```python
from build123d import *

# Parameters (mm, degrees)
SKETCH3_W           = 19.70074215
SKETCH3_H           = 14.68
SKETCH3_R           = 2
BOSS_EXTRUDE2_DEPTH = 4
SKETCH5_W           = 4
SKETCH5_H           = 14.68
BOSS_EXTRUDE3_DEPTH = 20
SKETCH6_R           = 2
CUT_EXTRUDE1_DEPTH  = 10
FILLET1_R           = 2


with BuildPart() as part:
    # Sketch3 → Boss-Extrude2 (new body)
    with BuildSketch(Plane(origin=(0, 0, 0), x_dir=(1, 0, 0), z_dir=(0, 1, 0))):
        with Locations((0.919743343, 1.910780827)):
            Rectangle(SKETCH3_W, SKETCH3_H)
        with Locations((1.919743345, 1.910780827)):
            Circle(SKETCH3_R, mode=Mode.SUBTRACT)
    extrude(amount=BOSS_EXTRUDE2_DEPTH)

    # Sketch5 → Boss-Extrude3 (add)
    with BuildSketch(Plane(origin=(0, 4, 0), x_dir=(1, 0, 0), z_dir=(0, 1, 0))):
        with Locations((-6.930627732, 1.910780827)):
            Rectangle(SKETCH5_W, SKETCH5_H)
    extrude(amount=BOSS_EXTRUDE3_DEPTH)

    # Sketch6 → Cut-Extrude1 (cut)
    with BuildSketch(Plane(origin=(-4.930627732, 0, 0), x_dir=(0, 0, -1), z_dir=(1, 0, 0))):
        with Locations((1.910780827, 14)):
            Circle(SKETCH6_R)
    extrude(amount=-CUT_EXTRUDE1_DEPTH, mode=Mode.SUBTRACT)

    # Fillet1
    fillet1_edges = [part.edges().sort_by_distance(p)[0] for p in [
        (-4.930627732, 4, -1.910780827),
        (-6.930627732, 24, 5.429219173),
        (-6.930627732, 24, -9.250780827),
        (10.770114418, 2, -9.250780827),
        (10.770114418, 2, 5.429219173),
    ]]
    fillet(fillet1_edges, radius=FILLET1_R)


solid = part.part
```
Build history of the part. All positions in model axes, mm. A direction names the side the tool comes from. Coordinates: 2 decimals unless noted, no trailing zeros. Order: outer loops, then holes, each group sorted by start corner. A loop starts at its lowest first (then second) coordinate and runs counter-clockwise, first axis right, second up. Notation, with made-up numbers: (-12, -14) -> (25, -14) arc R24 ccw to (25, 12) -> close; hole circle Ø11 at (4, -15). An arc over 180 degrees is marked (long way). Answer in a Markdown table with one row per item. Add a question column.
Q1. Mould opens along X. For faces 1 (the face through (1.486, 1.972, 0.042)), 2 (the face through (-8.931, 11.8, -1.8)), 3 (the face through (10.17, 2.03, -8.68)) say: +X half, -X half, draft (parallel to the pull), parting line (faces both ways), or undercut.
Q2. Band-saw the part on A-A, the plane y = 14. List the corners of the cut face in (x, z).
Q3. Drop flat-ended pins along their axis: pin 1 (7 mm diameter, centred on x = 6, z = -4, fed in from +Y); pin 2 (5 mm diameter, centred on y = 19.5, z = -2, fed in from +X). Give the stop position or say it passes through.
Q4. Wall check: line 1 along Y through (x, z) = (-2.25, 0); line 2 along X through (y, z) = (14.75, -8.25); line 3 along X through (y, z) = (4.75, -0.5). Give the ranges that are in metal, low to high. Write a range as [from, to].
Q5. Band-saw the part on B-B, the plane x = -5.5. List the corners of the cut face in (y, z), then the cut area to 3 significant figures.
Q6. Band-saw the part on C-C, the plane y = 3.5. List the corners of the cut face in (x, z).
Q7. Band-saw the part on D-D, the plane z = -2.25. List the corners of the cut face in (x, y).
Q8. Which spindle directions (+Z, -Z, +X, -X, +Y, -Y) get a long thin tool onto all of the face, cutting with end or side? Do faces 4 (the face through (-6.9, 23.43, 4.83)), 5 (the face through (-4.931, 17, -2)). Say none if no direction does.
Answers follow:
| question | item | result |
|---|---|---|
| 1 | face 1 | undercut |
| 1 | face 2 | -X half |
| 1 | face 3 | +X half |
| 2 | outline | (-8.93, -9.25) -> (-4.93, -9.25) -> (-4.93, -3.91) -> (-8.93, -3.91) -> close; (-8.93, 0.09) -> (-4.93, 0.09) -> (-4.93, 5.43) -> (-8.93, 5.43) -> close |
| 3 | pin 1 | y = 4 |
| 3 | pin 2 | x = -4.93 |
| 4 | line 1 | [0, 4] |
| 4 | line 2 | [-8.93, -4.93] |
| 4 | line 3 | [-8.93, -4.49] |
| 5 | outline | (0, -9.25) -> (22, -9.25) arc R2 ccw to (24, -7.25) -> (24, 3.43) arc R2 ccw to (22, 5.43) -> (0, 5.43) -> close; hole circle Ø4 at (14, -1.91) |
| 5 | area | 338 mm^2 |
| 6 | outline | (-8.93, -9.25) -> (8.77, -9.25) arc R2 ccw to (10.77, -7.25) -> (10.77, 3.43) arc R2 ccw to (8.77, 5.43) -> (-8.93, 5.43) -> close; hole circle Ø4 at (1.92, -1.91) |
| 7 | outline | (-8.93, 0) -> (-0.05, 0) -> (-0.05, 4) -> (-2.93, 4) arc R2 cw to (-4.93, 6) -> (-4.93, 12.03) -> (-8.93, 12.03) -> close; (-8.93, 15.97) -> (-4.93, 15.97) -> (-4.93, 24) -> (-8.93, 24) -> close; (3.89, 0) -> (10.77, 0) -> (10.77, 4) -> (3.89, 4) -> close |
| 8 | face 4 | +Z, +X, -X, +Y |
| 8 | face 5 | +Z, -Z, +X, +Y |
